from build123d import *

# Parameters (mm, degrees)
F0_R     = 75
F1_DEPTH = 50
F2_R     = 37.5
F3_DEPTH = 200
F4_R     = 55
F4_R_2   = 37.5
F5_DEPTH = 50
F6_R     = 12.5
F7_DEPTH = 50


with BuildPart() as f1:
    # F0 (on Top) → F1 (new body)
    with BuildSketch(Plane.XY):
        Circle(F0_R)
    extrude(amount=F1_DEPTH)

    # F2 (on face) → F3 (join)
    with BuildSketch(Plane.XY.offset(50)):
        Circle(F2_R)
    extrude(amount=F3_DEPTH)

    # F4 (on face) → F5 (join)
    with BuildSketch(Plane.XY.offset(250)):
        Circle(F4_R)
        Circle(F4_R_2, mode=Mode.SUBTRACT)
        Circle(F4_R_2)
    extrude(amount=F5_DEPTH)

    # F6 (on face) → F7 (join)
    with BuildSketch(Plane.XY.offset(300)):
        Circle(F6_R)
    extrude(amount=F7_DEPTH)


solid = f1.part
Read the model definition and answer for the solid it produces. Units are mm, in the model's axes. A direction names the side the tool comes from. Coordinates: 2 decimals unless noted, no trailing zeros. Write each loop counter-clockwise with the first axis right and the second up, starting at its lowest first coordinate (ties: lowest second). Pieces come first, ordered by that corner, then holes. Notation, with made-up numbers: (10.25, -10) -> (36.25, -10) arc R19 cw to (36.25, 1) -> close; hole circle Ø4 at (-2.75, 83). An arc over 180 degrees is marked (long way). Return JSON: item names as keys, results as strings.
(1) The part is cut by section A-A on x = 0. Give the vertices of the cut face in (y, z).
Answers below:
{"outline": "(-75, 0) -> (75, 0) -> (75, 50) -> (37.5, 50) -> (37.5, 250) -> (55, 250) -> (55, 300) -> (12.5, 300) -> (12.5, 350) -> (-12.5, 350) -> (-12.5, 300) -> (-55, 300) -> (-55, 250) -> (-37.5, 250) -> (-37.5, 50) -> (-75, 50) -> close"}
(2) For a pull along Z with two mould halves and no side action, classify faces 4 (the flat face through (15.6, 34.4, 50)), 5 (the flat face through (-1, 13, 300)), 6 (the cylindrical face through (-9.764, 74.362, 24.65)) as pulls with the +Z half, pulls with the -Z half, needs draft (parallel to the pull), parting line crosses it, or undercut.
Answers below:
{"face 4": "undercut", "face 5": "pulls with the +Z half", "face 6": "needs draft"}
(3) Which of the six approach directions +Z, -Z, +X, -X, +Y, -Y give full straight-line access (tool end or side, diameter ignored) to faces 1 (the cylindrical face through (11.923, 3.755, 324.65)), 2 (the flat face through (0, 0, 350)), 3 (the cylindrical face through (-4.88, 37.18, 148.6))?
Answers below:
{"face 1": "+Z", "face 2": "+Z, +X, -X, +Y, -Y", "face 3": "none"}
(4) The part is cut by section C-C on y = 49.5. Give the vertices of the cut face in (x, z), then the cut area to 3 significant figures.
Answers below:
{"outline": "(-56.34, 0) -> (56.34, 0) -> (56.34, 50) -> (-56.34, 50) -> close; (-23.97, 250) -> (23.97, 250) -> (23.97, 300) -> (-23.97, 300) -> close", "area": "8,030 mm^2"}
(5) Each of these flat-tipped pins is pushed along its axis until it touches: P1, Ø2, axis at x = 9.5, z = 241.5, coming from the -Y side; P2, Ø12, axis at y = -18.5, z = 249.5, coming from the +X side; P3, Ø5, axis at x = -41, y = -26.5, coming from the +Z side. Where does it stop, or does it pass through?
Answers below:
{"P1": "y = -36.52", "P2": "x = 53.56", "P3": "z = 300"}
(6) Consider line 1 along Z through (x, y) = (6, 48.5); line 2 along Z through (x, y) = (-6.5, -15); line 3 along X through (y, z) = (2, 40). Determine where each line is inside the solid, lowest interval first. Write a range as from..to.
Answers below:
{"line 1": "0..50, 250..300", "line 2": "0..300", "line 3": "-74.97..74.97"}
(7) The part is cut by section D-D on x = 45.5. Give the vertices of the cut face in (y, z), then the cut area to 3 significant figures.
Answers below:
{"outline": "(-59.62, 0) -> (59.62, 0) -> (59.62, 50) -> (-59.62, 50) -> close; (-30.9, 250) -> (30.9, 250) -> (30.9, 300) -> (-30.9, 300) -> close", "area": "9,050 mm^2"}
